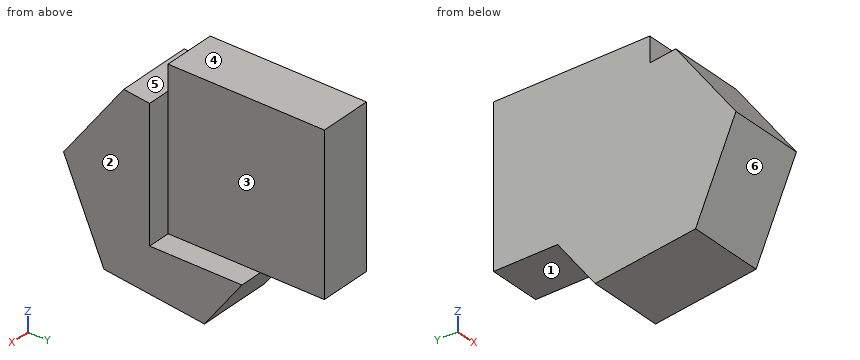
```python
from build123d import *

# Parameters (mm, degrees)
F4_DEPTH = 25
F6_DEPTH = 36


with BuildPart() as f4:
    # F2 (on Right) → F4 (new body)
    with BuildSketch(Plane.YZ):
        Polygon((23.118287, 0), (23.118287, 30.795261), (-50.702602, 30.795261), (-50.702602, 19.038247), (-50.702602, -43.253601), (-7.1146, -43.253601), (23.118287, -43.253601), align=None)
    extrude(amount=F4_DEPTH)

    # F1 (on face) → F6 (join)
    with BuildSketch(Plane.YZ):
        Polygon((-62.939021, 20.429226), (-91.347322, -17.983027), (-72.285485, -61.791464), (-24.815348, -67.187647), (-7.1146, -43.253601), (-50.702602, -43.253601), (-50.702602, 19.038247), align=None)
    extrude(amount=F6_DEPTH)


solid = f4.part
```
Could you check a few things on this model? Use its own coordinates, in mm. Face numbers are marked on the shaded views. A direction names the side the tool comes from. Round coordinates to 2 decimals unless told otherwise and drop trailing zeros. Write each loop counter-clockwise with the first axis right and the second up, starting at its lowest first coordinate (ties: lowest second). Pieces come first, ordered by that corner, then holes. Notation, with made-up numbers: M 1,83 L 17,83 A33 cw 17,113 Z; hole C 24.5,-31 d4. An arc over 180 degrees is marked long. Answer in a Markdown table with one row per item. Add a question column.
Q1. On a 3-axis mill with a long thin cutter (end or side, diameter ignored), from which of +Z, -Z, +X, -X, +Y, -Y can I reach the whole of each face in a straight line? I mean the marked faces 1, 2 and 3. Say none if no direction works.
Q2. Imagine slicing it at B-B (z = 23). Please give me the cut outline in (x, y), then the cut area to 3 significant figures.
Q3. Imagine slicing it at D-D (z = -9). Please give me the cut outline in (x, y).
Q4. If I drill on line 1 (X direction, y = 9.5, z = -38); line 2 (Z direction, x = 8, y = 14); line 3 (Y direction, x = 29, z = -51.5), over which ranges is the centre line in solid material (lowest first)? Write a range as from..to.
Q5. Imagine slicing it at A-A (x = 29). Please give me the cut outline in (y, z), then the cut area to 3 significant figures.
Q6. If we mould it in two halves opening along Y, with no side actions, what happens to the marked faces 4, 5 and 6? For each: +Y half, -Y half, draft (parallel to the pull), parting line (faces both ways), or undercut.
Q7. Will these pins go through, and if not, where does the flat tip stop? pin 1 Ø10 at (x, z) = (29.5, -51) entering from +Y; pin 2 Ø12 at (x, y) = (31.5, -33) entering from +Z; pin 3 Ø12 at (x, z) = (27, 0.5) entering from -Y.
Q8. Imagine slicing it at C-C (y = -34.5). Please give me the cut outline in (x, z), then the cut area to 3 significant figures.
Values:
| question | item | result |
|---|---|---|
| 1 | face 1 | -Z, +X, -X, +Y |
| 1 | face 2 | +Z, -Z, +X, +Y, -Y |
| 1 | face 3 | +Z, +X, +Y |
| 2 | outline | M 0,-50.7 L 25,-50.7 L 25,23.12 L 0,23.12 Z |
| 2 | area | 1,850 mm^2 |
| 3 | outline | M 0,-84.7 L 36,-84.7 L 36,-50.7 L 25,-50.7 L 25,23.12 L 0,23.12 Z |
| 4 | line 1 | 0..25 |
| 4 | line 2 | -43.25..30.8 |
| 4 | line 3 | -76.76..-13.21 |
| 5 | outline | M -91.35,-17.98 L -72.29,-61.79 L -24.82,-67.19 L -7.11,-43.25 L -50.7,-43.25 L -50.7,19.04 L -62.94,20.43 Z |
| 5 | area | 3,190 mm^2 |
| 6 | face 4 | draft |
| 6 | face 5 | undercut |
| 6 | face 6 | -Y half |
| 7 | pin 1 | y = -9.15 |
| 7 | pin 2 | z = -43.25 |
| 7 | pin 3 | y = -82.12 |
| 8 | outline | M 0,-66.09 L 36,-66.09 L 36,-43.25 L 25,-43.25 L 25,30.8 L 0,30.8 Z |
| 8 | area | 2,670 mm^2 |
